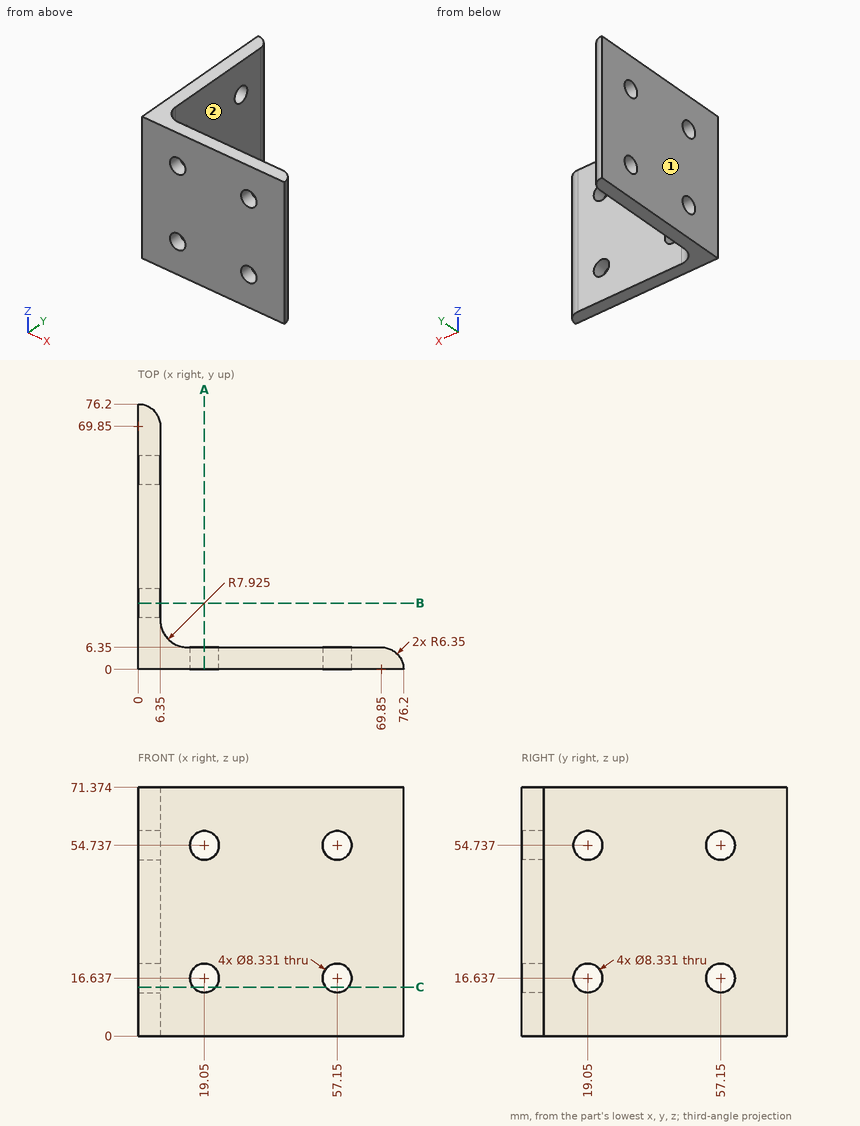
Study the drawing (mm; zero at the part's minimum x, y, z) and answer. A direction names the side the tool comes from. Give positions to 0.01 mm unless a question says otherwise; leave off trailing zeros. Loops run counter-clockwise (first coordinate to the right, second up) from the corner with the lowest first, then second, coordinate; pieces in that order, holes last. Notation, with made-up numbers: M 28,79 L 61,79 A12 cw 61,94 Z; hole C -20,16 d5. An arc over 180 degrees is marked long. One line per item, written item: value. Start each with the question number.
1. Each of these flat-tipped pins is pushed along its axis until it touches: P1, Ø6, axis at x = 27, z = 52.5, coming from the +Y side; P2, Ø11, axis at y = 57.15, z = 16.637, coming from the +X side. Where does it stop, or does it pass through?
2. Find section C-C (z = 14). State how many separate pieces and enclosed holes the cut face has, and give its area (3 significant figures).
3. Find section A-A (x = 19.05). Give the vertices of the cut face in (y, z), and give its area (3 significant figures).
4. Find the intervals of material crossed by probe 1 along Z at (x, y) = (4, 57); probe 2 along X at (y, z) = (3, 54); probe 3 along Y at (x, z) = (28, 35), in increasing order.
5. Which of the six approach directions +Z, -Z, +X, -X, +Y, -Y give full straight-line access (tool end or side, diameter ignored) to the marked faces 1 and 2?
Reported:
1. P1: stops at y = 6.35
1. P2: stops at x = 6.35
2. separate pieces: 5
2. enclosed holes: 0
2. area: 760 mm²
3. outline: M 0,0 L 6.35,0 L 6.35,12.47 L 0,12.47 Z; M 0,20.8 L 6.35,20.8 L 6.35,50.57 L 0,50.57 Z; M 0,58.9 L 6.35,58.9 L 6.35,71.37 L 0,71.37 Z
3. area: 347 mm²
4. probe 1: z = 0 to 12.47, 20.8 to 50.57, 58.9 to 71.37
4. probe 2: x = 0 to 14.95, 23.15 to 53.05, 61.25 to 75.45
4. probe 3: y = 0 to 6.35
5. face 1: +Z, -Z, -X, +Y, -Y
5. face 2: +Z, -Z, +X, +Y
